```python
from build123d import *

# Parameters (mm, degrees)
BOSS_EXTRUDE1_DEPTH = 469.9
SKETCH2_W           = 10.16
SKETCH2_H           = 83.810703233
SKETCH2_H_2         = 111.159792755
SKETCH2_H_3         = 83.757510526
SKETCH2_H_4         = 83.784106879
SKETCH2_H_5         = 83.730914172
SKETCH2_H_6         = 83.704317819
SKETCH2_H_7         = 83.677721465
SKETCH2_H_8         = 83.651125112
SKETCH2_H_9         = 22.104476438
CUT_EXTRUDE1_DEPTH  = 10.16
SKETCH3_W           = 10.16
SKETCH3_H           = 55.879999965
SKETCH3_H_2         = 88.9
SKETCH3_H_3         = 109.22
CUT_EXTRUDE2_DEPTH  = 12.7
SKETCH4_W           = 81.316938584
SKETCH4_H           = 20.32
SKETCH4_W_2         = 81.316938585
CUT_EXTRUDE3_DEPTH  = 12.7
SKETCH5_W           = 89.916
SKETCH5_H           = 20.32
CUT_EXTRUDE4_DEPTH  = 12.7
CUT_EXTRUDE5_DEPTH  = 137.414
SKETCH13_R          = 3.175
CUT_EXTRUDE8_DEPTH  = 2128.667464702
CUT_EXTRUDE9_DEPTH  = 2128.667464702
SKETCH20_R          = 4.7625
CUT_EXTRUDE10_DEPTH = 2107.728843747
SKETCH24_R          = 3.175
CUT_EXTRUDE12_DEPTH = 12.7


with BuildPart() as part:
    # Sketch1 → Boss-Extrude1 (new body)
    with BuildSketch(Plane.XY):
        Polygon((-215.881789204, 2052.32), (-215.881789204, 1463.040000035), (-316.088635901, 20.32), (-317.499999939, 0), (-307.333509538, 0), (-205.715298803, 1463.040000035), (-205.715298803, 2072.64), (-215.881789204, 2072.64), align=None)
    extrude(amount=-BOSS_EXTRUDE1_DEPTH)

    # Sketch2 → Cut-Extrude1 (cut)
    with BuildSketch(Plane(origin=(-315.975651309, 21.946686571, 0), x_dir=(0, 0, 1), z_dir=(-0.9975965627192115, 0.06928995634877068, 0))):
        with Locations((-5.08, 247.132760087)):
            Rectangle(SKETCH2_W, SKETCH2_H)
        with Locations((-5.08, 55.684811679)):
            Rectangle(SKETCH2_W, SKETCH2_H_2)
        with Locations((-5.08, 602.706163733)):
            Rectangle(SKETCH2_W, SKETCH2_H_3)
        with Locations((-5.08, 424.91946191)):
            Rectangle(SKETCH2_W, SKETCH2_H_4)
        with Locations((-5.08, 780.492865556)):
            Rectangle(SKETCH2_W, SKETCH2_H_5)
        with Locations((-5.08, 958.27956738)):
            Rectangle(SKETCH2_W, SKETCH2_H_6)
        with Locations((-5.08, 1136.066269203)):
            Rectangle(SKETCH2_W, SKETCH2_H_7)
        with Locations((-5.08, 1313.852971026)):
            Rectangle(SKETCH2_W, SKETCH2_H_8)
        with Locations((-5.08, -10.947322918)):
            Rectangle(SKETCH2_W, SKETCH2_H_9)
        with Locations((-464.82, -10.947322918)):
            Rectangle(SKETCH2_W, SKETCH2_H_9)
        with Locations((-464.82, 55.684811679)):
            Rectangle(SKETCH2_W, SKETCH2_H_2)
        with Locations((-464.82, 247.132760087)):
            Rectangle(SKETCH2_W, SKETCH2_H)
        with Locations((-464.82, 424.91946191)):
            Rectangle(SKETCH2_W, SKETCH2_H_4)
        with Locations((-464.82, 602.706163733)):
            Rectangle(SKETCH2_W, SKETCH2_H_3)
        with Locations((-464.82, 780.492865556)):
            Rectangle(SKETCH2_W, SKETCH2_H_5)
        with Locations((-464.82, 958.27956738)):
            Rectangle(SKETCH2_W, SKETCH2_H_6)
        with Locations((-464.82, 1136.066269203)):
            Rectangle(SKETCH2_W, SKETCH2_H_7)
        with Locations((-464.82, 1313.852971026)):
            Rectangle(SKETCH2_W, SKETCH2_H_8)
    extrude(amount=-CUT_EXTRUDE1_DEPTH, mode=Mode.SUBTRACT)

    # Sketch3 → Cut-Extrude2 (cut)
    with BuildSketch(Plane.ZY.offset(215.881789204)):
        with Locations((-5.08, 1490.980000018)):
            Rectangle(SKETCH3_W, SKETCH3_H)
        with Locations((-5.08, 1652.27)):
            Rectangle(SKETCH3_W, SKETCH3_H_2)
        Polygon((-469.9, 1463.040000035), (-459.713026258, 1463.040000035), (-453.620872406, 1546.589538567), (-463.753970086, 1547.328410273), (-457.607940173, 1631.616820512), (-447.474842492, 1630.877948806), (-441.328812579, 1715.166359045), (-451.461910259, 1715.905230751), (-445.315880346, 1800.19364099), (-435.182782665, 1799.454769284), (-429.036752752, 1883.743179522), (-439.169850432, 1884.482051228), (-433.023820518, 1968.770461467), (-422.890722838, 1968.031589761), (-415.263026258, 2072.64), (-469.9, 2072.64), align=None)
        with Locations((-5.08, 1830.07)):
            Rectangle(SKETCH3_W, SKETCH3_H_2)
        with Locations((-5.08, 2018.03)):
            Rectangle(SKETCH3_W, SKETCH3_H_3)
    extrude(amount=-CUT_EXTRUDE2_DEPTH, mode=Mode.SUBTRACT)

    # Sketch4 → Cut-Extrude3 (cut)
    with BuildSketch(Plane.ZY.offset(215.881789204)):
        with Locations((-376.086223632, 2062.48)):
            Rectangle(SKETCH4_W, SKETCH4_H)
        with Locations((-213.452346463, 2062.48)):
            Rectangle(SKETCH4_W_2, SKETCH4_H)
        with Locations((-50.818469292, 2062.48)):
            Rectangle(SKETCH4_W_2, SKETCH4_H)
    extrude(amount=-CUT_EXTRUDE3_DEPTH, mode=Mode.SUBTRACT)

    # Sketch5 → Cut-Extrude4 (cut)
    with BuildSketch(Plane(origin=(-315.975651309, 21.946686571, 0), x_dir=(0, 0, 1), z_dir=(-0.9975965627192115, 0.06928995634877068, 0))):
        with Locations((-414.782, -11.839561137)):
            Rectangle(SKETCH5_W, SKETCH5_H)
        with Locations((-234.95, -11.839561137)):
            Rectangle(SKETCH5_W, SKETCH5_H)
        with Locations((-55.118, -11.839561137)):
            Rectangle(SKETCH5_W, SKETCH5_H)
    extrude(amount=-CUT_EXTRUDE4_DEPTH, mode=Mode.SUBTRACT)

    # Sketch6 → Cut-Extrude5 (cut)
    with BuildSketch(Plane(origin=(-315.975651309, 21.946686571, 0), x_dir=(0, 0, 1), z_dir=(-0.9975965627192115, 0.06928995634877068, 0))):
        Polygon((-87.26775037, 725.157981502), (-65.68812669, 678.917255627), (-74.89887104, 674.61878511), (-96.478494721, 720.859510985), align=None)
        Polygon((-53.31924736, 628.378059234), (-44.10850301, 632.676529752), (-22.52887933, 586.435803877), (-31.73962368, 582.137333359), align=None)
        Polygon((-117.688081031, 364.457321541), (-109.500847052, 358.426570287), (-55.568463259, 431.644155721), (-63.755697238, 437.674906975), align=None)
        Polygon((-225.552848619, 218.022150673), (-217.372552167, 211.996509631), (-163.440168374, 285.214095065), (-171.620464825, 291.239736107), align=None)
        Polygon((-333.417616206, 71.586979805), (-325.230382227, 65.556228551), (-271.297998434, 138.773813985), (-279.485232413, 144.804565239), align=None)
    extrude(amount=-CUT_EXTRUDE5_DEPTH, mode=Mode.SUBTRACT)

    # Sketch13 → Cut-Extrude8 (cut, through all)
    with BuildSketch(Plane.ZY.offset(215.881789204)):
        with Locations(Location((-25.246459893, 1731.87, 0), (0, 0, 270))):
            Circle(SKETCH13_R)
        with Locations(Location((-70.408959893, 1755.42, 0), (0, 0, 270))):
            Circle(SKETCH13_R)
        with Locations(Location((-182.408959893, 1755.42, 0), (0, 0, 270))):
            Circle(SKETCH13_R)
        with Locations(Location((-25.246459893, 1918.97, 0), (0, 0, 270))):
            Circle(SKETCH13_R)
        with Locations(Location((-47.788959893, 1865.42, 0), (0, 0, 270))):
            Circle(SKETCH13_R)
        with Locations(Location((-182.408959893, 1910.42, 0), (0, 0, 270))):
            Circle(SKETCH13_R)
        with Locations(Location((-117.078959893, 1910.42, 0), (0, 0, 270))):
            Circle(SKETCH13_R)
        with Locations(Location((-70.408959893, 1895.42, 0), (0, 0, 270))):
            Circle(SKETCH13_R)
        with Locations(Location((-317.028959893, 1865.42, 0), (0, 0, 270))):
            Circle(SKETCH13_R)
        with Locations(Location((-294.408959893, 1755.42, 0), (0, 0, 270))):
            Circle(SKETCH13_R)
        with Locations(Location((-317.028959893, 1785.42, 0), (0, 0, 270))):
            Circle(SKETCH13_R)
        with Locations(Location((-339.571459893, 1731.87, 0), (0, 0, 270))):
            Circle(SKETCH13_R)
        with Locations(Location((-339.571459893, 1918.97, 0), (0, 0, 270))):
            Circle(SKETCH13_R)
    extrude(amount=-CUT_EXTRUDE8_DEPTH, mode=Mode.SUBTRACT)

    # Sketch17 → Cut-Extrude9 (cut, through all)
    with BuildSketch(Plane.ZY.offset(215.881789204)):
        Polygon((-91.602336227, 1471.504269383), (-81.702736369, 1473.789772095), (-94.643375784, 1529.841839519), (-104.542975642, 1527.556336807), align=None)
        Polygon((-130.424254473, 1639.660471655), (-117.483615058, 1583.608404231), (-107.584015199, 1585.893906943), (-120.524654614, 1641.945974367), align=None)
    extrude(amount=-CUT_EXTRUDE9_DEPTH, mode=Mode.SUBTRACT)

    # Sketch20 → Cut-Extrude10 (cut, through all)
    with BuildSketch(Plane(origin=(-315.975651309, 21.946686571, 0), x_dir=(0, 0, 1), z_dir=(-0.9975965627192116, 0.06928995634876853, 0))):
        with Locations(Location((-35.56, 347.287639338, 0), (0, 0, 270))):
            Circle(SKETCH20_R)
        with Locations(Location((-35.56, 302.837639338, 0), (0, 0, 270))):
            Circle(SKETCH20_R)
        Polygon((-120.929306778, 445.712379572), (-154.823537638, 399.698212032), (-162.492565561, 405.347250509), (-128.598334701, 451.361418049), align=None)
    extrude(amount=-CUT_EXTRUDE10_DEPTH, mode=Mode.SUBTRACT)

    # Sketch24 → Cut-Extrude12 (cut)
    with BuildSketch(Plane.ZY.offset(215.881789204)):
        with Locations(Location((-39.313746491, 1670.454214013, 0), (0, 0, 270))):
            Circle(SKETCH24_R)
    extrude(amount=-CUT_EXTRUDE12_DEPTH, mode=Mode.SUBTRACT)


solid = part.part
```
Build history of the part. All positions in model axes, mm. A direction names the side the tool comes from. Round coordinates to 2 decimals unless told otherwise and drop trailing zeros.
1) 3-axis set-ups, long thin cutter, end or side, ignore diameter. For faces 1 (the flat face through (-303.46, 130.05, -306.07)), 2 (the flat face through (-215.882, 1772, -229)), 3 (the flat face through (-303.94, 123.01, -298.64)): which of +Z, -Z, +X, -X, +Y, -Y reach the whole face in a straight line?
2) Drill centre lines: probe 1 along Z at (x, y) = (-209, 1865.42); probe 2 along Z at (x, y) = (-211, 1910); probe 3 along X at (y, z) = (1865, -365). Where is each one in solid material? Low to high.
3) Pin check, flat tips, straight feed: pin 1 (9 mm diameter, centred on x = -312.5, y = 11.5, fed in from -Z); pin 2 (3 mm diameter, centred on y = 494.5, z = -236.5, fed in from -X); pin 3 (3 mm diameter, centred on y = 761.5, z = -96, fed in from -X); pin 4 (4 mm diameter, centred on y = 1865.42, z = -317.03, fed in from -X). Stop position of each tip, or through.
4) Mould opens along Y. For faces 4 (the flat face through (-257.236, 721.279, -231.661)), 5 (the flat face through (-283.651, 415.175, -82.912)), 6 (the flat face through (-205.715, 1764, -229)) say: +Y half, -Y half, draft (parallel to the pull), parting line (faces both ways), or undercut.
Ans:
1. face 1: -X
1. face 2: +Z, -Z, -X, +Y
1. face 3: +X
2. probe 1: z = -430.37 to -320.2, -313.85 to -50.96, -44.61 to -10.16
2. probe 2: z = -437.31 to -185.56, -179.26 to -120.23, -113.93 to 0
2. probe 3: x = -215.88 to -205.72
3. pin 1: stops at z = -369.82
3. pin 2: stops at x = -283.26
3. pin 3: stops at x = -264.71
3. pin 4: passes through
4. face 4: -Y half
4. face 5: undercut
4. face 6: draft
